```python
from build123d import *

# Parameters (mm, degrees)
SKETCH1_R               = 40.005
SKETCH1_R_2             = 38.1
BOSS_EXTRUDE1_DEPTH     = 3.175
SKETCH1_3_R             = 38.1
BOSS_EXTRUDE2_DEPTH     = 12.7
CUT_EXTRUDE1_DEPTH      = 59.760664351
CUT_EXTRUDE1_DEPTH_BACK = 59.760664351
SKETCH3_R               = 2.4892
CUT_EXTRUDE2_DEPTH      = 59.760664351
CUT_EXTRUDE2_DEPTH_BACK = 59.760664351
SKETCH4_R               = 2.4892
BOSS_EXTRUDE3_START     = 8.89
SKETCH4_3_R             = 4.445
SKETCH4_3_R_2           = 2.4892
BOSS_EXTRUDE3_DEPTH     = 8.89
FILLET1_R               = 2.54


with BuildPart() as part:
    # Sketch1 → Boss-Extrude1 (new body)
    # profile 1 of 2: a face of its own
    with BuildSketch(Plane(origin=(0, 0, 0), x_dir=(1, 0, 0), z_dir=(0, 1, 0))):
        with Locations(Location((0, 0, 0), (0, 0, 270))):
            Circle(SKETCH1_R)
        Circle(SKETCH1_R_2, mode=Mode.SUBTRACT)
    # profile 2 of 2: a face of its own
    with BuildSketch(Plane(origin=(0, 0, 0), x_dir=(1, 0, 0), z_dir=(0, 1, 0))):
        Circle(SKETCH1_R_2)
    extrude(amount=BOSS_EXTRUDE1_DEPTH)

    # Sketch1_3 → Boss-Extrude2 (add)
    with BuildSketch(Plane(origin=(0, 0, 0), x_dir=(1, 0, 0), z_dir=(0, 1, 0))):
        with Locations(Location((0, 0, 0), (0, 0, 270))):
            Circle(SKETCH1_3_R)
    extrude(amount=-BOSS_EXTRUDE2_DEPTH)

    # Sketch3 → Cut-Extrude1 (cut, two sides: drawn at the far end of the back side and taken through both)
    with BuildSketch(Plane(origin=(0, 3.175, 0), x_dir=(1, 0, 0), z_dir=(0, 1, 0)).offset(-CUT_EXTRUDE1_DEPTH_BACK)):
        with Locations(Location((-25.015, 0, 0), (0, 0, 270))):
            Circle(SKETCH3_R)
        with Locations(Location((25.015, 0, 0), (0, 0, 270))):
            Circle(SKETCH3_R)
    extrude(amount=CUT_EXTRUDE1_DEPTH + CUT_EXTRUDE1_DEPTH_BACK, mode=Mode.SUBTRACT)

    # Sketch4 → Cut-Extrude2 (cut, two sides: drawn at the far end of the back side and taken through both)
    with BuildSketch(Plane(origin=(0, 3.175, 0), x_dir=(1, 0, 0), z_dir=(0, 1, 0)).offset(-CUT_EXTRUDE2_DEPTH_BACK)):
        with Locations(Location((-16.389946669, -23.407269666, 0), (0, 0, 270))):
            Circle(SKETCH4_R)
        with Locations(Location((16.389946669, 23.407269666, 0), (0, 0, 270))):
            Circle(SKETCH4_R)
    extrude(amount=CUT_EXTRUDE2_DEPTH + CUT_EXTRUDE2_DEPTH_BACK, mode=Mode.SUBTRACT)

    # Sketch4_3 → Boss-Extrude3 (add)
    # profile 1 of 2: a face of its own
    with BuildSketch(Plane(origin=(0, 3.175, 0), x_dir=(1, 0, 0), z_dir=(0, 1, 0)).offset(BOSS_EXTRUDE3_START)):
        with Locations(Location((16.389946669, 23.407269666, 0), (0, 0, 270))):
            Circle(SKETCH4_3_R)
        with Locations(Location((16.389946669, 23.407269666, 0), (0, 0, 270))):
            Circle(SKETCH4_3_R_2, mode=Mode.SUBTRACT)
    # profile 2 of 2: a face of its own
    with BuildSketch(Plane(origin=(0, 3.175, 0), x_dir=(1, 0, 0), z_dir=(0, 1, 0)).offset(BOSS_EXTRUDE3_START)):
        with Locations(Location((-16.389946669, -23.407269666, 0), (0, 0, 90))):
            Circle(SKETCH4_3_R)
        with Locations(Location((-16.389946669, -23.407269666, 0), (0, 0, 270))):
            Circle(SKETCH4_3_R_2, mode=Mode.SUBTRACT)
    extrude(amount=-BOSS_EXTRUDE3_DEPTH)

    # Fillet1
    fillet1_edges = [part.edges().sort_by_distance(p)[0] for p in [
        (16.389946669, 3.175, -27.852269666),
        (-16.389946669, 3.175, 27.852269666),
    ]]
    fillet(fillet1_edges, radius=FILLET1_R)


solid = part.part
```
Part model, mm, in its own coordinate system. A direction names the side the tool comes from. Round coordinates to 2 decimals unless told otherwise and drop trailing zeros. Write each loop counter-clockwise with the first axis right and the second up, starting at its lowest first coordinate (ties: lowest second). Pieces come first, ordered by that corner, then holes. Notation, with made-up numbers: (-20, 5) -> (25, 5) arc R22 cw to (25, 32) -> close; hole circle Ø6 at (86, 30.5). An arc over 180 degrees is marked (long way). Return JSON: item names as keys, results as strings. Group by question number.
Q1. Saw through at C-C on y = -6.5. Write the cut outline in (x, z) (3 decimals).
Q2. Saw through at A-A on z = 0. Write the cut outline in (x, y) (3 decimals).
Q3. Saw through at B-B on x = -3.5. Write the cut outline in (y, z) (3 decimals).
Q4. Mould opens along X. For faces 1 (the cylindrical face through (12.016, 1.565, 38.158)), 2 (the cylindrical face through (-22.547, -4.874, -0.324)), 3 (the flat face through (-14, 12.065, 21)) say: pulls with the +X half, pulls with the -X half, needs draft (parallel to the pull), parting line crosses it, or undercut.
Q5. Probe L1, parallel to Y at x = -22.5, z = -27 (3 decimals); L2, parallel to Z at x = -27, y = -9; L3, parallel to Z at x = 15, y = -3.5. List the from-to ranges inside material, lowest first. Write a range as [from, to].
Q6. Pin check, flat tips, straight feed: pin 1 (1.5 mm diameter, centred on y = 1.5, z = -8.5, fed in from -X); pin 2 (4 mm diameter, centred on y = 0, z = -19, fed in from +X); pin 3 (4 mm diameter, centred on x = -20, y = -5.5, fed in from -Z). Stop position of each tip, or through.
Q7. Which spindle directions (+Z, -Z, +X, -X, +Y, -Y) get a long thin tool onto all of the face, cutting with end or side? Do faces 4 (the cylindrical face through (-23.183, -6.261, -30.235)), 5 (the flat face through (14, 12.065, -21)), 6 (the cylindrical face through (-17.73, 8.93, 19.17)). Say none if no direction does.
Q8. Saw through at D-D on z = -32. Write the cut outline in (x, y) (3 decimals).
Answer:
{
 "1": {"outline": "circle Ø76.2 at (0, 0); hole circle Ø4.978 at (-25.015, 0); hole circle Ø4.978 at (-16.39, 23.407); hole circle Ø4.978 at (16.39, -23.407); hole circle Ø4.978 at (25.015, 0)"},
 "2": {"outline": "(-40.005, 0) -> (-38.1, 0) -> (-38.1, -12.7) -> (-27.504, -12.7) -> (-27.504, 3.175) -> (-40.005, 3.175) -> close; (-22.526, -12.7) -> (22.526, -12.7) -> (22.526, 3.175) -> (-22.526, 3.175) -> close; (27.504, -12.7) -> (38.1, -12.7) -> (38.1, 0) -> (40.005, 0) -> (40.005, 3.175) -> (27.504, 3.175) -> close"},
 "3": {"outline": "(-12.7, -37.939) -> (0, -37.939) -> (0, -39.852) -> (3.175, -39.852) -> (3.175, 39.852) -> (0, 39.852) -> (0, 37.939) -> (-12.7, 37.939) -> close"},
 "4": {"face 1": "parting line crosses it", "face 2": "undercut", "face 3": "needs draft"},
 "5": {"L1": "[-12.7, 3.175]", "L2": "[-26.88, -1.5], [1.5, 26.88]", "L3": "[-35.02, -25.47], [-21.34, 35.02]"},
 "6": {"pin 1": "x = -39.25", "pin 2": "x = 36.21", "pin 3": "z = -33.58"},
 "7": {"face 4": "-Y", "face 5": "+Z, -Z, +X, -X, +Y", "face 6": "+Y"},
 "8": {"outline": "(-24.008, 0) -> (-20.679, 0) -> (-20.679, -12.7) -> (20.679, -12.7) -> (20.679, 0) -> (24.008, 0) -> (24.008, 3.175) -> (-24.008, 3.175) -> close"}
}
